Source: CAD feature listing. Evaluate the final solid. Frame: model axes, mm. A direction names the side the tool comes from. Give positions to 0.01 mm unless a question says otherwise; leave off trailing zeros. Loops run counter-clockwise (first coordinate to the right, second up) from the corner with the lowest first, then second, coordinate; pieces in that order, holes last. Notation, with made-up numbers: (2, 47.25) - (50, 47.25) arc R25 ccw to (50, 74.25) - close; hole circle Ø10 at (18.25, 21.5). An arc over 180 degrees is marked (long way). Put each result on its own line as item: value.
```python
from build123d import *

# Parameters (mm, degrees)
EXTRUDE_1_DEPTH    = 20
EXTRUDE_2_DEPTH    = 25
HOLE_WIZARD_M5_1_D = 4.2
HOLE_WIZARD_M5_2_D = 4.2


with BuildPart() as part:
    # 草图1 → 凸台-拉伸1 (new body)
    with BuildSketch(Plane(origin=(0, 0, 0), x_dir=(1, 0, 0), z_dir=(0, 1, 0))):
        Polygon((-3, 3), (-3, -3), (-1, -5), (1.2, -5), (1.2, -3), (3, -3), (3, 3), (1.2, 3), (1.2, 5), (-1, 5), align=None)
    extrude(amount=EXTRUDE_1_DEPTH)

    # 草图3 → 凸台-拉伸2 (add)
    with BuildSketch(Plane.ZY.offset(3)):
        Polygon((-3, -6), (3, -6), (5, -4), (5, -1.8), (3, -1.8), (3, 0), (-3, 0), (-3, -1.8), (-5, -1.8), (-5, -4), align=None)
    extrude(amount=-EXTRUDE_2_DEPTH)

    # M5 螺纹孔1 (through all)
    with Locations(Plane.ZY.offset(3)):
        with Locations((0, 10)):
            Hole(HOLE_WIZARD_M5_1_D / 2)

    # M5 螺纹孔2 (through all)
    with Locations(Plane(origin=(0, -6, 0), x_dir=(-1, 0, 0), z_dir=(0, -1, 0))):
        with Locations((-12, 0)):
            Hole(HOLE_WIZARD_M5_2_D / 2)


solid = part.part
```
1) Section query B-B, the plane z = -3.75. Output: boundary loops of the cut face in (x, y), plus the area to 3 significant figures.
Check result:
outline: (-3, -5.25) - (22, -5.25) - (22, -1.8) - (-3, -1.8) - close; (-2.25, 0) - (1.2, 0) - (1.2, 20) - (-2.25, 20) - close
area: 155 mm²
2) Mould query, pull axis X, two halves, no side actions, for faces 6 (the flat face through (-2, 10, -4)), 7 (the flat face through (0, 0, 4)), 8 (the cylindrical face through (9.9, -2.96, -0.09)). Classes: pulls with the +X half, pulls with the -X half, needs draft (parallel to the pull), parting line crosses it, or undercut.
Check result:
face 6: pulls with the -X half
face 7: needs draft
face 8: undercut
3) Section query C-C, the plane x = 12. Output: boundary loops of the cut face in (y, z).
Check result:
outline: (-6, -3) - (-4, -5) - (-1.8, -5) - (-1.8, -3) - (0, -3) - (0, -2.1) - (-6, -2.1) - close; (-6, 2.1) - (0, 2.1) - (0, 3) - (-1.8, 3) - (-1.8, 5) - (-4, 5) - (-6, 3) - close
4) Section query A-A, the plane y = 10. Output: boundary loops of the cut face in (x, z).
Check result:
outline: (-3, -3) - (-1, -5) - (1.2, -5) - (1.2, -3) - (3, -3) - (3, -2.1) - (-3, -2.1) - close; (-3, 2.1) - (3, 2.1) - (3, 3) - (1.2, 3) - (1.2, 5) - (-1, 5) - (-3, 3) - close
5) Section query D-D, the plane z = 1.5. Output: boundary loops of the cut face in (x, y).
Check result:
outline: (-3, -6) - (10.53, -6) - (10.53, 0) - (3, 0) - (3, 8.53) - (-3, 8.53) - close; (-3, 11.47) - (3, 11.47) - (3, 20) - (-3, 20) - close; (13.47, -6) - (22, -6) - (22, 0) - (13.47, 0) - close
6) Pin query (flat end, axial travel): P1, Ø1, axis at x = -1.5, z = 4, coming from the -Y side; P2, Ø1, axis at x = 9, z = -4, coming from the +Y side; P3, Ø3, axis at x = 13, z = -1, coming from the +Y side. Return the tip coordinate at first contact, or that it passes through.
Check result:
P1: y = -5.5
P2: y = -1.8
P3: y = 0
7) Access query for faces 1 (the flat face through (-2, 10, 4)), 2 (the flat face through (9, -3, 5)), 3 (the flat face through (9, -1.8, -4)), 4 (the flat face through (1.2, 10, 4)), 5 (the flat face through (3, 7.6, 0)). Directions: +Z, -Z, +X, -X, +Y, -Y. A direction counts if a zero-diameter tool reaches every point of the face in a straight line with its end or side. Return the directions, or none.
Check result:
face 1: +Z, -X, +Y
face 2: +Z, +X, -X, +Y, -Y
face 3: -Z, +X, -X
face 4: +Z, +X, +Y
face 5: +Z, -Z, +X, +Y
8) Material intervals for line 1 along Y through (x, z) = (0.85, 0); line 2 along Z through (x, y) = (12, -2.05); line 3 along X through (y, z) = (15, -1.25), sorted ascending. Write a range as [from, to].
Check result:
line 1: [-6, 7.9], [12.1, 20]
line 2: [-5, -2.1], [2.1, 5]
line 3: [-3, 3]
